Source: CAD feature listing. Evaluate the final solid. Frame: model axes, mm. Face numbers are marked on the shaded views. A direction names the side the tool comes from. Round coordinates to 2 decimals unless told otherwise and drop trailing zeros. Order: outer loops, then holes, each group sorted by start corner. A loop starts at its lowest first (then second) coordinate and runs counter-clockwise, first axis right, second up. Notation, with made-up numbers: (56, -20) -> (106, -20) arc R27 ccw to (106, 13) -> close; hole circle Ø6 at (78, 36.25). An arc over 180 degrees is marked (long way). Write item = value, one per line. Start each with the question number.
(1) Reachability of the marked faces 4, 5, 6 and 7 from +Z, -Z, +X, -X, +Y, -Y: full face, straight path, thin tool, end or side. Return the list, or none.
(2) Cut plane C-C on x = -10. Return the cut outline in (y, z), then the cut area to 3 significant figures.
(3) Contact query for flat-ended pins moving along their axis: pin 1 Ø22 at (x, z) = (193, 15) entering from +Y; pin 2 Ø10 at (x, y) = (112.5, -23) entering from -Z; pin 3 Ø8 at (x, z) = (134.5, -36) entering from -Y. Output: stop coordinate, or through.
(4) Draft query along X for the marked faces 1, 2 and 3. Return one class per face: released by +X, released by -X, zero draft, split by the parting line, or undercut.
(5) Ray query, line 1 (X direction, y = -57.5, z = -71.5); line 2 (Z direction, x = 74.5, y = 20); line 3 (Y direction, x = 129, z = -34). Return the intervals inside material, ascending.
(6) Cut plane B-B on z = -36. Return the cut outline in (x, y).
(7) Cut plane D-D on z = -49.5. Return the cut outline in (x, y), then the cut area to 3 significant figures.
(8) Cut plane A-A on y = -55. Return the cut outline in (x, z), then the cut area to 3 significant figures.
from build123d import *

# Parameters (mm, degrees)
IZIM1_W                          = 280
IZIM1_H                          = 100
IZIM1_W_2                        = 240
IZIM1_H_2                        = 60
Y_KSEKLIK_EKSTR_ZYON1_DEPTH      = 30
IZIM2_R                          = 7.5
Y_KSEKLIK_EKSTR_ZYON2_DEPTH      = 70
IZIM4_R                          = 11
KES_EKSTR_ZYON1_DEPTH            = 40
IZIM5_W                          = 65
IZIM5_H                          = 15
KES_EKSTR_ZYON2_DEPTH            = 119
KES_EKSTR_ZYON3_DEPTH            = 24.5
Y_KSEKLIK_EKSTR_ZYON4_DEPTH      = 8
Y_KSEKLIK_EKSTR_ZYON4_DEPTH_BACK = 1
IZIM13_R                         = 7.75
KES_EKSTR_ZYON4_DEPTH            = 18


with BuildPart() as part:
    # Çizim1 → Yükseklik-Ekstrüzyon1 (new body)
    with BuildSketch(Plane(origin=(0, 0, 0), x_dir=(1, 0, 0), z_dir=(0, 1, 0))):
        with Locations((120, 30)):
            Rectangle(IZIM1_W, IZIM1_H)
        with Locations((120, 30)):
            Rectangle(IZIM1_W_2, IZIM1_H_2, mode=Mode.SUBTRACT)
    extrude(amount=Y_KSEKLIK_EKSTR_ZYON1_DEPTH)

    # Çizim2 → Yükseklik-Ekstrüzyon2 (add)
    with BuildSketch(Plane(origin=(0, 0, 0), x_dir=(-1, 0, 0), z_dir=(0, -1, 0))):
        with Locations(Location((10, -10, 0), (0, 0, 90))):
            Circle(IZIM2_R)
        with Locations(Location((-250, -10, 0), (0, 0, 270))):
            Circle(IZIM2_R)
        with Locations(Location((10, 70, 0), (0, 0, 270))):
            Circle(IZIM2_R)
        with Locations(Location((-250, 70, 0), (0, 0, 90))):
            Circle(IZIM2_R)
        with Locations(Location((-120, -10, 0), (0, 0, 90))):
            Circle(IZIM2_R)
        with Locations(Location((-120, 70, 0), (0, 0, 90))):
            Circle(IZIM2_R)
    extrude(amount=Y_KSEKLIK_EKSTR_ZYON2_DEPTH)

    # Çizim4 → Kes-Ekstrüzyon1 (cut, symmetric)
    with BuildSketch(Plane.XY.offset(-30)):
        with Locations((228.036930768, 15)):
            Circle(IZIM4_R)
        with Locations((16.579541137, 15)):
            Circle(IZIM4_R)
        with Locations((95.469880506, 15)):
            Circle(IZIM4_R)
    extrude(amount=KES_EKSTR_ZYON1_DEPTH, both=True, mode=Mode.SUBTRACT)

    # Çizim5 → Kes-Ekstrüzyon2 (cut)
    with BuildSketch(Plane.XY.offset(20)):
        with Locations((177.478221097, 22.5)):
            Rectangle(IZIM5_W, IZIM5_H)
    extrude(amount=-KES_EKSTR_ZYON2_DEPTH, mode=Mode.SUBTRACT)

    # Çizim6 → Kes-Ekstrüzyon3 (cut, symmetric)
    with BuildSketch(Plane.XY.offset(-30)):
        Polygon((260, 31.552276972), (234.133246527, 31.552276972), (234.359911555, 20.467639669), (260, 4.801073138), align=None)
    extrude(amount=KES_EKSTR_ZYON3_DEPTH, both=True, mode=Mode.SUBTRACT)

    # Çizim10 → Yükseklik-Ekstrüzyon4 (add, two sides: drawn at the far end of the back side and taken through both)
    with BuildSketch(Plane(origin=(0, 22, 0), x_dir=(1, 0, 0), z_dir=(0, 1, 0)).offset(-Y_KSEKLIK_EKSTR_ZYON4_DEPTH_BACK)):
        Polygon((55.057032044, 60), (144.978221097, 21.175943648), (144.978221097, 60), align=None)
    extrude(amount=Y_KSEKLIK_EKSTR_ZYON4_DEPTH + Y_KSEKLIK_EKSTR_ZYON4_DEPTH_BACK)

    # Çizim13 → Kes-Ekstrüzyon4 (cut)
    with BuildSketch(Plane(origin=(0, 0, -80), x_dir=(-1, 0, 0), z_dir=(0, 0, -1))):
        with Locations((-16.579541137, 15)):
            Circle(IZIM13_R)
    extrude(amount=-KES_EKSTR_ZYON4_DEPTH, mode=Mode.SUBTRACT)


solid = part.part
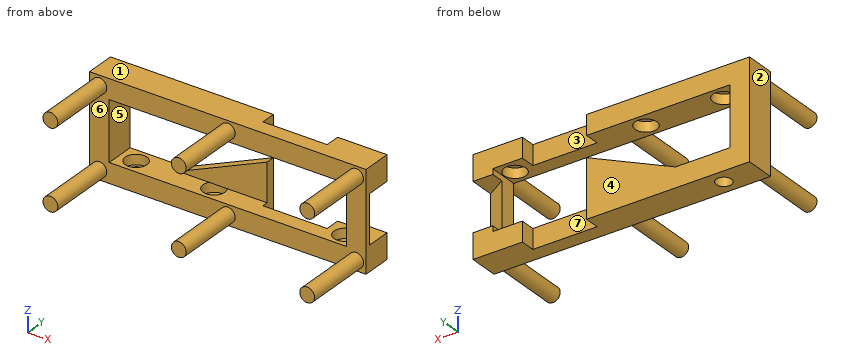
Evaluation:
q1.face_4 = +Z, -Z, +X, -X, +Y
q1.face_5 = +Y, -Y
q1.face_6 = -Y
q1.face_7 = +Z, -Z, +Y
q2.outline = (-70, -77.5) -> (0, -77.5) -> (0, -80) -> (30, -80) -> (30, 20) -> (0, 20) -> (0, 17.5) -> (-70, 17.5) -> (-70, 2.5) -> (0, 2.5) -> (0, -62.5) -> (-70, -62.5) -> close
q2.area = 5,100 mm^2
q3.pin_1 = 15
q3.pin_2 = -77.07
q3.pin_3 = 21
q4.face_1 = zero draft
q4.face_2 = released by -X
q4.face_3 = undercut
q5.line_1 = -17.35 to -2.65, 112.65 to 127.35, 242.65 to 257.35
q5.line_2 = -80 to -60, 0 to 20
q5.line_3 = 21 to 30
q6.outline = (-20, 0) -> (0, 0) -> (0, 30) -> (-20, 30) -> close; (110.64, 21) -> (144.98, 21) -> (144.98, 30) -> (110.64, 30) -> close; (240, 0) -> (260, 0) -> (260, 4.8) -> (240, 17.02) -> close
q7.outline = (-20, 0) -> (0, 0) -> (0, 30) -> (-20, 30) -> close; (79.38, 21) -> (144.98, 21) -> (144.98, 30) -> (79.38, 30) -> close; (240, 0) -> (260, 0) -> (260, 4.8) -> (240, 17.02) -> close
q7.area = 1,410 mm^2
q8.outline = circle Ø15 at (-10, -70); circle Ø15 at (-10, 10); circle Ø15 at (120, -70); circle Ø15 at (120, 10); circle Ø15 at (250, -70); circle Ø15 at (250, 10)
q8.area = 1,060 mm^2
